The listing builds one solid part. Answer for the finished solid, in the listing's coordinates (mm). Face numbers are marked on the shaded views. A direction names the side the tool comes from. Coordinates: 2 decimals unless noted, no trailing zeros. Loops run counter-clockwise (first coordinate to the right, second up) from the corner with the lowest first, then second, coordinate; pieces in that order, holes last. Notation, with made-up numbers: M 36,71 L 80,71 A30 ccw 80,103 Z; hole C 77,22 d5. An arc over 180 degrees is marked long. Return JSON: item names as keys, results as strings. Group by question number.
1. Section B-B (y = 0) is taken. Write down the section's boundary in (x, z).
2. The mould has two halves that part along X. Classify the marked faces 1, 2, 3 and 4: pulls with the +X half, pulls with the -X half, needs draft (parallel to the pull), parting line crosses it, or undercut.
3. Section C-C (z = 4) is taken. Write down the section's boundary in (x, y).
4. Section A-A (x = 0) is taken. Write down the section's boundary in (y, z).
5. Given P1, Ø6, axis at x = 16, y = -2.5, coming from the +Z side; P2, Ø5, axis at x = -5.5, z = 6, coming from the -Y side; P3, Ø1, axis at x = -6.5, z = 8, coming from the +Y side, each flat-ended and moving along its own axis, determine where each tip first touches the part or whether it passes through.
6. Section D-D (y = 7.75) is taken. Write down the section's boundary in (x, z), then the cut area to 3 significant figures.
7. Which of the six approach directions +Z, -Z, +X, -X, +Y, -Y give full straight-line access (tool end or side, diameter ignored) to the marked faces 5 and 6?
8. Straight lines are drawn through the part: L1, parallel to Y at x = 0, z = 5.25; L2, parallel to Z at x = 14.5, y = -4; L3, parallel to Y at x = 16, z = 0.9. For each, find the intervals that lie inside material, in ascending order. Write a range as from..to.
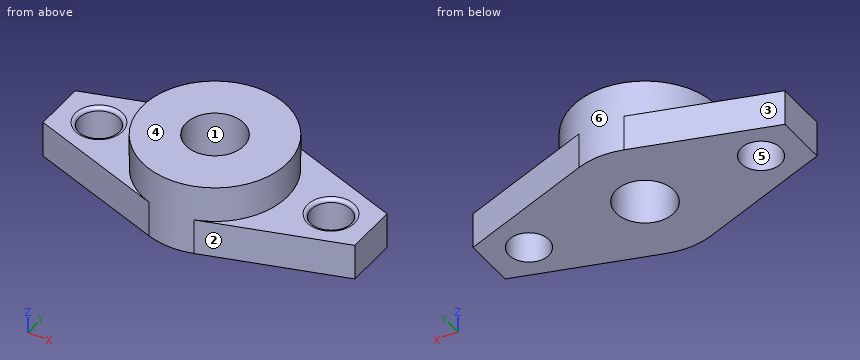
```python
from build123d import *

# Parameters (mm, degrees)
SKETCH_1_R        = 2.75
EXTRUDE_1_DEPTH   = 5
EXTRUDE_1_2_DEPTH = 5
SKETCH_2_R        = 10
SKETCH_2_R_2      = 4
EXTRUDE_2_DEPTH   = 10
FILLET_2_R        = 0.5
FILLET_3_R        = 0.5


with BuildPart() as part:
    # Sketch 1 → Extrude 1 (new body)
    with BuildSketch(Plane.XY):
        with BuildLine():
            Line((21.5, 3.5), (3.10364576, 9.506176045))
            ThreePointArc((3.10364576, 9.506176045), (8.094333129, 5.872118119), (10, 0))
            ThreePointArc((10, 0), (8.094333129, -5.872118119), (3.10364576, -9.506176045))
            Line((3.10364576, -9.506176045), (21.5, -3.5))
            Line((21.5, -3.5), (21.5, 3.5))
        make_face()
        with Locations((16, 0)):
            Circle(SKETCH_1_R, mode=Mode.SUBTRACT)
    extrude(amount=EXTRUDE_1_DEPTH)



with BuildPart() as body_2:
    # Sketch 1 → Extrude 1 2 (new body)
    with BuildSketch(Plane.XY):
        with BuildLine():
            Line((-3.10364576, 9.506176045), (-21.5, 3.5))
            Line((-21.5, 3.5), (-21.5, -3.5))
            Line((-21.5, -3.5), (-3.10364576, -9.506176045))
            ThreePointArc((-3.10364576, -9.506176045), (-10, 0), (-3.10364576, 9.506176045))
        make_face()
        with Locations((-16, 0)):
            Circle(SKETCH_1_R, mode=Mode.SUBTRACT)
    extrude(amount=EXTRUDE_1_2_DEPTH)


with BuildPart() as part_1:
    add(part.part)

    add(body_2.part)  # Extrude 2 merges body 2
    # Sketch 2 → Extrude 2 (add)
    with BuildSketch(Plane.XY):
        with Locations(Location((0, 0, 0), (0, 0, 108.081202901))):
            Circle(SKETCH_2_R)
        Circle(SKETCH_2_R_2, mode=Mode.SUBTRACT)
    extrude(amount=EXTRUDE_2_DEPTH)

    # Fillet 2
    fillet_2_edges = [part_1.edges().sort_by_distance(p)[0] for p in [
        (-18.75, 0, 5),
    ]]
    fillet(fillet_2_edges, radius=FILLET_2_R)

    # Fillet 3
    fillet_3_edges = [part_1.edges().sort_by_distance(p)[0] for p in [
        (13.25, 0, 5),
    ]]
    fillet(fillet_3_edges, radius=FILLET_3_R)


solid = part_1.part
```
Worked out:
{
 "1": {"outline": "M -21.5,0 L -18.75,0 L -18.75,4.5 A0.5 ccw -19.25,5 L -21.5,5 Z; M -13.25,0 L -4,0 L -4,10 L -10,10 L -10,5 L -12.75,5 A0.5 ccw -13.25,4.5 Z; M 4,0 L 13.25,0 L 13.25,4.5 A0.5 ccw 12.75,5 L 10,5 L 10,10 L 4,10 Z; M 18.75,0 L 21.5,0 L 21.5,5 L 19.25,5 A0.5 ccw 18.75,4.5 Z"},
 "2": {"face 1": "undercut", "face 2": "pulls with the +X half", "face 3": "pulls with the -X half", "face 4": "needs draft"},
 "3": {"outline": "M -21.5,-3.5 L -3.1,-9.51 A10 ccw 3.1,-9.51 L 21.5,-3.5 L 21.5,3.5 L 3.1,9.51 A10 ccw -3.1,9.51 L -21.5,3.5 Z; hole C -16,0 d5.5; hole C 0,0 d8; hole C 16,0 d5.5"},
 "4": {"outline": "M -10,0 L -4,0 L -4,10 L -10,10 Z; M 4,0 L 10,0 L 10,10 L 4,10 Z"},
 "5": {"P1": "z = 5", "P2": "y = -9.54", "P3": "y = 8"},
 "6": {"outline": "M -8.48,0 L 8.48,0 L 8.48,5 L 6.32,5 L 6.32,10 L -6.32,10 L -6.32,5 L -8.48,5 Z", "area": "148 mm^2"},
 "7": {"face 5": "+Z, -Z", "face 6": "+Z"},
 "8": {"L1": "-10..-4, 4..10", "L2": "0..5", "L3": "-5.3..-2.75, 2.75..5.3"}
}
